Read the model definition and answer for the solid it produces. Units are mm, in the model's axes. A direction names the side the tool comes from. Round coordinates to 2 decimals unless told otherwise and drop trailing zeros. Loops run counter-clockwise (first coordinate to the right, second up) from the corner with the lowest first, then second, coordinate; pieces in that order, holes last. Notation, with made-up numbers: (62.25, -31) -> (99.25, -31) arc R15 cw to (99.25, -22) -> close; hole circle Ø1 at (82.25, 49). An arc over 180 degrees is marked (long way). Put each result on its own line as item: value.
from build123d import *

# Parameters (mm, degrees)
SKETCH1_W           = 41
SKETCH1_H           = 16
BOSS_EXTRUDE1_DEPTH = 3
SKETCH2_W           = 45
SKETCH2_H           = 20
SKETCH2_W_2         = 41
SKETCH2_H_2         = 16
BOSS_EXTRUDE2_DEPTH = 7


with BuildPart() as part:
    # Sketch1 → Boss-Extrude1 (new body)
    with BuildSketch(Plane(origin=(0, 0, 0), x_dir=(1, 0, 0), z_dir=(0, 1, 0))):
        Rectangle(SKETCH1_W, SKETCH1_H)
    extrude(amount=BOSS_EXTRUDE1_DEPTH)

    # Sketch2 → Boss-Extrude2 (add)
    with BuildSketch(Plane.XZ):
        Rectangle(SKETCH2_W, SKETCH2_H)
        Rectangle(SKETCH2_W_2, SKETCH2_H_2, mode=Mode.SUBTRACT)
    extrude(amount=-BOSS_EXTRUDE2_DEPTH)


solid = part.part
Item 1: The part is cut by section B-B (y = 6). Determine the outline of the cut face in (x, z).
Derived:
outline: (-22.5, -10) -> (22.5, -10) -> (22.5, 10) -> (-22.5, 10) -> close; hole (-20.5, -8) -> (20.5, -8) -> (20.5, 8) -> (-20.5, 8) -> close
Item 2: Which of the six approach directions +Z, -Z, +X, -X, +Y, -Y give full straight-line access (tool end or side, diameter ignored) to faces 5 (the flat face through (0, 3, -10)), 6 (the flat face through (0, 5, -8))?
Derived:
face 5: -Z, +X, -X, +Y, -Y
face 6: +Y
Item 3: The part is cut by section C-C (z = 5). Determine the outline of the cut face in (x, y).
Derived:
outline: (-22.5, 0) -> (22.5, 0) -> (22.5, 7) -> (20.5, 7) -> (20.5, 3) -> (-20.5, 3) -> (-20.5, 7) -> (-22.5, 7) -> close
Item 4: Find the intervals of material crossed by line 1 along X through (y, z) = (4.5, -6.25); line 2 along Z through (x, y) = (4.5, 4.25); line 3 along Y through (x, z) = (-18.5, 3.5), in increasing order.
Derived:
line 1: x = -22.5 to -20.5, 20.5 to 22.5
line 2: z = -10 to -8, 8 to 10
line 3: y = 0 to 3
Item 5: For a pull along X with two mould halves and no side action, classify faces 1 (the flat face through (22.5, 3, 0)), 2 (the flat face through (-20.5, 5, 0)), 3 (the flat face through (0, 3, 10)), 4 (the flat face through (0, 3, 0)) as pulls with the +X half, pulls with the -X half, needs draft (parallel to the pull), parting line crosses it, or undercut.
Derived:
face 1: pulls with the +X half
face 2: undercut
face 3: needs draft
face 4: undercut
Item 6: The part is cut by section A-A (x = -12.5). Determine the outline of the cut face in (y, z), then the cut area to 3 significant figures.
Derived:
outline: (0, -10) -> (7, -10) -> (7, -8) -> (3, -8) -> (3, 8) -> (7, 8) -> (7, 10) -> (0, 10) -> close
area: 76.0 mm^2
Item 7: A flat-ended cylindrical pin translates along its axis: pin 1 Ø4 at (x, z) = (0, -2) entering from +Y. Find the tip coordinate at first contact, or state that the pin passes through.
Derived:
pin 1: stops at y = 3
